Input: part model. Units: mm. Frame: model coordinates. A direction names the side the tool comes from. Give positions to 0.01 mm unless a question says otherwise; leave off trailing zeros. Write each loop counter-clockwise with the first axis right and the second up, starting at its lowest first coordinate (ties: lowest second). Pieces come first, ordered by that corner, then holes. Notation, with made-up numbers: (-20, 13.5) -> (9, 13.5) arc R4 cw to (9, 18.5) -> close; hole circle Ø4 at (73.5, -27). An arc over 180 degrees is marked (long way). Answer as a JSON object with one key per item and string values. Group by question number.
from build123d import *

# Parameters (mm, degrees)
F1_DEPTH = 5.5
F0_R     = 1.5
F2_DEPTH = 3
F3_R     = 1.5
F4_DEPTH = 1


with BuildPart() as f1:
    # F0 (on Front) → F1 (new body)
    with BuildSketch(Plane.XZ):
        with BuildLine():
            ThreePointArc((9.4391472072, 1.75), (0, 9.6), (-9.4391472072, 1.75))
            Line((-9.4391472072, 1.75), (-8.215686216, 1.75))
            ThreePointArc((-8.215686216, 1.75), (0, 8.4), (8.215686216, 1.75))
            Line((8.215686216, 1.75), (9.4391472072, 1.75))
        make_face()
    extrude(amount=F1_DEPTH)



with BuildPart() as f1b:
    # F0 (on Front) → F1, piece 2 (new body)
    with BuildSketch(Plane.XZ):
        with BuildLine():
            Line((-8.215686216, -1.75), (-9.4391472072, -1.75))
            ThreePointArc((-9.4391472072, -1.75), (0, -9.6), (9.4391472072, -1.75))
            Line((9.4391472072, -1.75), (8.215686216, -1.75))
            ThreePointArc((8.215686216, -1.75), (0, -8.4), (-8.215686216, -1.75))
        make_face()
    extrude(amount=F1_DEPTH)


with BuildPart() as f1_1:
    add(f1.part)

    add(f1b.part)  # F2 merges F1b
    # F0 (on Front) → F2 (join)
    with BuildSketch(Plane.XZ):
        with BuildLine():
            Line((8.215686216, -1.75), (9.4391472072, -1.75))
            ThreePointArc((9.4391472072, -1.75), (9.6, 0), (9.4391472072, 1.75))
            Line((9.4391472072, 1.75), (8.215686216, 1.75))
            ThreePointArc((8.215686216, 1.75), (8.3537944736, 0.8798396972), (8.4, 0))
            ThreePointArc((8.4, 0), (8.3537944736, -0.8798396972), (8.215686216, -1.75))
        make_face()
        with BuildLine():
            ThreePointArc((-9.4391472072, 1.75), (-9.6, 0), (-9.4391472072, -1.75))
            Line((-9.4391472072, -1.75), (-8.215686216, -1.75))
            ThreePointArc((-8.215686216, -1.75), (-8.4, 0), (-8.215686216, 1.75))
            Line((-8.215686216, 1.75), (-9.4391472072, 1.75))
        make_face()
        with BuildLine():
            ThreePointArc((-8.215686216, 1.75), (-8.4, 0), (-8.215686216, -1.75))
            ThreePointArc((-8.215686216, -1.75), (0, -8.4), (8.215686216, -1.75))
            ThreePointArc((8.215686216, -1.75), (8.3537944736, -0.8798396972), (8.4, 0))
            ThreePointArc((8.4, 0), (8.3537944736, 0.8798396972), (8.215686216, 1.75))
            ThreePointArc((8.215686216, 1.75), (0, 8.4), (-8.215686216, 1.75))
        make_face()
        Circle(F0_R, mode=Mode.SUBTRACT)
    extrude(amount=F2_DEPTH)

    # F3 (on face) → F4 (cut)
    with BuildSketch(Plane.XZ.offset(3)):
        Polygon((1.6454482672, -2.85), (3.2908965344, 0), (1.6454482672, 2.85), (-1.6454482672, 2.85), (-3.2908965344, 0), (-1.6454482672, -2.85), align=None)
        Circle(F3_R, mode=Mode.SUBTRACT)
    extrude(amount=-F4_DEPTH, mode=Mode.SUBTRACT)


solid = f1_1.part
1. Section C-C (z = -1). Return the cut outline in (x, y), plus the area to 3 significant figures.
2. Reachability of faces 1 (the face through (-2, -2, 0)), 2 (the face through (0, 0, -2)), 3 (the face through (-9, -4, -1.75)) from +Z, -Z, +X, -X, +Y, -Y: full face, straight path, thin tool, end or side. Return the list, or none.
3. Section A-A (y = -4.9). Return the cut outline in (x, z).
4. Section D-D (x = 3). Return the cut outline in (y, z).
5. Contact query for flat-ended pins moving along their axis: pin 1 Ø1.7 at (x, z) = (1.5, 0) entering from -Y; pin 2 Ø0.6 at (x, y) = (-9, -5) entering from -Z; pin 3 Ø3 at (y, z) = (-3, 5.5) entering from +X. Output: stop coordinate, or through.
6. Section B-B (x = 0). Return the cut outline in (y, z), plus the area to 3 significant figures.
7. Mould query, pull axis Z, two halves, no side actions, for faces 4 (the face through (2.48, -2.507, 1.405)), 5 (the face through (-1, -5.5, 9)). Classes: pulls with the +Z half, pulls with the -Z half, needs draft (parallel to the pull), parting line crosses it, or undercut.
8. Line query: line 1 (Z direction, x = 0, y = -1.4); line 2 (Z direction, x = 0, y = -2.8); line 3 (Y direction, x = -0.25, z = -1.75). Output: solid intervals per line, ascending.
Working result:
{
 "1": {"outline": "(-9.55, -3) -> (-2.71, -3) -> (-2.71, -2) -> (-1.12, -2) -> (-1.12, 0) -> (-9.55, 0) -> close; (1.12, -2) -> (2.71, -2) -> (2.71, -3) -> (9.55, -3) -> (9.55, 0) -> (1.12, 0) -> close", "area": "47.4 mm^2"},
 "2": {"face 1": "-Y", "face 2": "+Z, -Z, +X, -X, +Y", "face 3": "+X, -X, -Y"},
 "3": {"outline": "(-9.44, -1.75) arc R9.6 ccw to (9.44, -1.75) -> (8.22, -1.75) arc R8.4 cw to (-8.22, -1.75) -> close; (-9.44, 1.75) -> (-8.22, 1.75) arc R8.4 cw to (8.22, 1.75) -> (9.44, 1.75) arc R9.6 ccw to start"},
 "4": {"outline": "(-5.5, -9.12) -> (0, -9.12) -> (0, 9.12) -> (-5.5, 9.12) -> (-5.5, 7.85) -> (-3, 7.85) -> (-3, 0.5) -> (-2, 0.5) -> (-2, -0.5) -> (-3, -0.5) -> (-3, -7.85) -> (-5.5, -7.85) -> close"},
 "5": {"pin 1": "stops at y = -2", "pin 2": "stops at z = -4.06", "pin 3": "stops at x = 8.73"},
 "6": {"outline": "(-5.5, -9.6) -> (0, -9.6) -> (0, -1.5) -> (-2, -1.5) -> (-2, -2.85) -> (-3, -2.85) -> (-3, -8.4) -> (-5.5, -8.4) -> close; (-5.5, 8.4) -> (-3, 8.4) -> (-3, 2.85) -> (-2, 2.85) -> (-2, 1.5) -> (0, 1.5) -> (0, 9.6) -> (-5.5, 9.6) -> close", "area": "51.9 mm^2"},
 "7": {"face 4": "undercut", "face 5": "needs draft"},
 "8": {"line 1": "z = -9.6 to -1.5, 1.5 to 9.6", "line 2": "z = -9.6 to -2.85, 2.85 to 9.6", "line 3": "y = -2 to 0"}
}
